Work out the finished part from the listing and answer in its coordinate system (mm). Coordinates: 2 decimals unless noted, no trailing zeros. Loops run counter-clockwise (first coordinate to the right, second up) from the corner with the lowest first, then second, coordinate; pieces in that order, holes last. Notation, with made-up numbers: (59.5, -14.75) -> (117.5, -14.75) arc R3 ccw to (117.5, -9.75) -> close; hole circle Ø9 at (17, 27.5). An arc over 180 degrees is marked (long way). Answer as CSV lines item,"result".
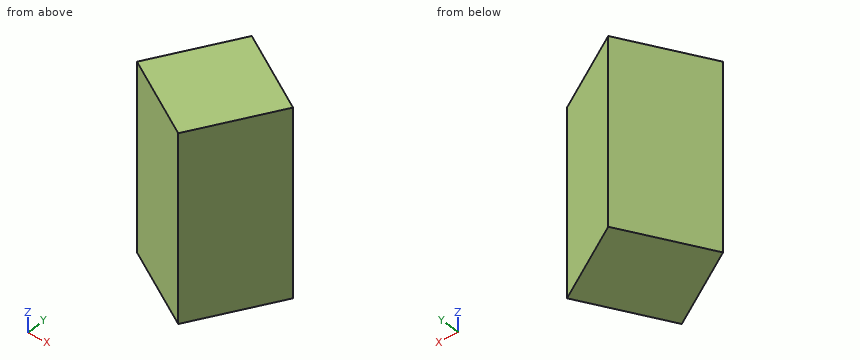
```python
from build123d import *

# Parameters (mm, degrees)
F1_DEPTH = 100
F2_DEPTH = 8.961
F3_DEPTH = 8.961
F4_DEPTH = 8.961


with BuildPart() as f1:
    # F0 (on Top) → F1 (new body)
    with BuildSketch(Plane.XY):
        Polygon((-10.6803802773, 40.3006346896), (-40.3006346896, -10.6803802773), (10.6803802773, -40.3006346896), (40.3006346896, 10.6803802773), align=None)
    extrude(amount=F1_DEPTH)

    # F2 (add): a face of the model
    f2_faces = [f1.faces().sort_by_distance(p)[0] for p in [
        (-25.4905074835, 14.8101272061, 50),
    ]]
    extrude(f2_faces, amount=-F2_DEPTH)

    # F3 (cut): a face of the model
    f3_faces = [f1.faces().sort_by_distance(p)[0] for p in [
        (-25.4905074835, 14.8101272061, 50),
    ]]
    extrude(f3_faces, amount=-F3_DEPTH, mode=Mode.SUBTRACT)

    # F4 (cut): a face of the model
    f4_faces = [f1.faces().sort_by_distance(p)[0] for p in [
        (-10.9360468067, -27.7413698313, 50),
    ]]
    extrude(f4_faces, amount=-F4_DEPTH, mode=Mode.SUBTRACT)


solid = f1.part
```
(1) A cutting plane is placed at A-A, the plane x = 34. Write down the section's boundary in (y, z), and give its area (3 significant figures).
Computed values:
outline,"(-0.16, 0) -> (14.34, 0) -> (14.34, 100) -> (-0.16, 100) -> close"
area,"1,450 mm2"
(2) A cutting plane is placed at B-B, the plane z = 81. Write down the section's boundary in (x, y).
Computed values:
outline,"(-28.05, -7.43) -> (15.18, -32.55) -> (40.3, 10.68) -> (-2.93, 35.8) -> close"
(3) Flat-ended cylindrical pins translate along their axes: pin 1 Ø10 at (x, z) = (13, 88.5) entering from -Y; pin 2 Ø1 at (x, z) = (26, 71.5) entering from +Y; pin 3 Ø5 at (x, z) = (20, 49.5) entering from -Y. Find the tip coordinate at first contact, or state that the pin passes through.
Computed values:
pin 1,"y = -32.55"
pin 2,"y = 19.28"
pin 3,"y = -28.56"
(4) Consider line 1 along Y through (x, z) = (-10, 63); line 2 along Y through (x, z) = (-11, 25); line 3 along X through (y, z) = (-27, 26). Determine where each line is inside the solid, lowest interval first.
Computed values:
line 1,"-17.92 to 23.63"
line 2,"-17.34 to 21.91"
line 3,"5.63 to 18.41"
